```python
from build123d import *

# Parameters (mm, degrees)
F0_W     = 75.6683796644
F0_H     = 56.6312596202
F1_DEPTH = 76.2
F2_R     = 32.8805478482
F2_R_2   = 27.3422805509
F2_R_3   = 19.1504254532
F2_R_4   = 11.9146478849
F3_DEPTH = 25.4
F4_R     = 25.8365396263
F4_R_2   = 16.7772933898
F4_R_3   = 9.0542222029
F5_DEPTH = 25.4
F6_T     = -2.54
F7_R     = 3.661512341
F7_R_2   = 9.1001332581
F7_R_3   = 2.6513181401
F7_R_4   = 8.8835137034
F7_R_5   = 3.3715323173
F7_R_6   = 9.593089253
F7_R_7   = 4.4394708986
F7_R_8   = 7.7443328278
F7_R_9   = 7.7443291059
F8_DEPTH = 25.4


with BuildPart() as f1:
    # F0 (on Front) → F1 (new body)
    with BuildSketch(Plane.XZ):
        with Locations((37.8341898322, 28.3156298101)):
            Rectangle(F0_W, F0_H)
    extrude(amount=F1_DEPTH)

    # F2 (on face) → F3 (join)
    with BuildSketch(Plane.XY.offset(56.6312596202)):
        with Locations((41.328176856, -39.9102717638)):
            Circle(F2_R)
        with Locations((41.328176856, -39.9102717638)):
            Circle(F2_R_2, mode=Mode.SUBTRACT)
        with Locations((41.328176856, -39.9102717638)):
            Circle(F2_R_2)
        with Locations((41.328176856, -39.9102717638)):
            Circle(F2_R_3, mode=Mode.SUBTRACT)
        with Locations((41.328176856, -39.9102717638)):
            Circle(F2_R_4)
    extrude(amount=F3_DEPTH)

    # F4 (on face) → F5 (join)
    with BuildSketch(Plane(origin=(0, 0, 0), x_dir=(0, -1, 0), z_dir=(-1, 0, 0))):
        with Locations((38.5897643864, 28.854271397)):
            Circle(F4_R)
        with Locations((38.5897643864, 28.854271397)):
            Circle(F4_R_2, mode=Mode.SUBTRACT)
        with Locations((38.5897643864, 28.854271397)):
            Circle(F4_R_2)
        with Locations((38.5897643864, 28.854271397)):
            Circle(F4_R_3, mode=Mode.SUBTRACT)
        with Locations((38.5897643864, 28.854271397)):
            Circle(F4_R_3)
    extrude(amount=F5_DEPTH)

    # F6
    f6_openings = [f1.faces().sort_by_distance(p)[0] for p in [
        (37.83419, -76.2, 28.31563),
    ]]
    offset(amount=F6_T, openings=f6_openings, kind=Kind.INTERSECTION)

    # F7 (on face) → F8 (join)
    with BuildSketch(Plane.YZ.offset(75.6683796644)):
        with Locations((-8.7984241545, 43.9281985164)):
            Circle(F7_R)
        with Locations((-25.612493977, 40.552649647)):
            Circle(F7_R_2)
        with Locations((-40.1582121849, 43.9281985164)):
            Circle(F7_R_3)
        with Locations((-42.6249019802, 32.3069766164)):
            Circle(F7_R_4)
        with Locations((-43.8523180783, 17.5502598286)):
            Circle(F7_R_5)
        with Locations((-27.9581807554, 16.7665481567)):
            Circle(F7_R_6)
        with Locations((-15.7014150172, 29.2281731963)):
            Circle(F7_R_7)
        with BuildLine():
            Line((0, 7.6459474177), (0, 12.9123390406))
            ThreePointArc((0, 12.9123390406), (-10.0560886873, 10.2791432291), (0, 7.6459474177))
        make_face()
        with Locations((-64.4422322512, 47.1135601401)):
            Circle(F7_R_8)
        with Locations((-64.5220428705, 12.6286838204)):
            Circle(F7_R_9)
    extrude(amount=F8_DEPTH)


solid = f1.part
```
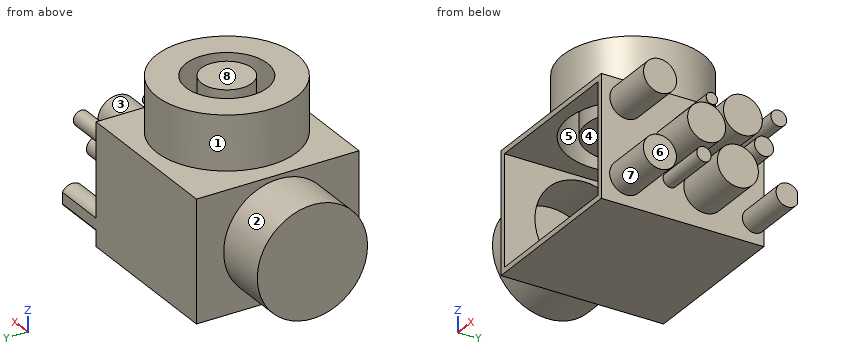
Model file for the job. Use its own axes, mm. Face numbers are marked on the shaded views. A direction names the side the tool comes from. Coordinates: 2 decimals unless noted, no trailing zeros. Loops run counter-clockwise (first coordinate to the right, second up) from the corner with the lowest first, then second, coordinate; pieces in that order, holes last. Notation, with made-up numbers: (57.5, -36) - (99.5, -36) arc R17 cw to (99.5, -10) - close; hole circle Ø7 at (-22, -1.5). An arc over 180 degrees is marked (long way). Answer as a JSON object with one key per item and string values. Group by question number.
(1) Tool access for the marked faces 1, 2, 3, 4 and 5: list every direction of +Z, -Z, +X, -X, +Y, -Y with a clear straight run to the whole face (end or side of a thin tool).
(2) Probe line 1 along X through (y, z) = (-47.5, 45.5); line 2 along X through (y, z) = (-20.5, 77); line 3 along Z through (x, y) = (43.5, -35.5). List the from-to ranges inside material, lowest first.
(3) Cut at D-D (z = 36.5). Give the cut face in (x, y).
(4) Flat gauge pins, fed straight in: pin 1 (12 mm diameter, centred on x = 68, y = -59.5, fed in from -Z); pin 2 (5 mm diameter, centred on x = 1, y = -45, fed in from +Z); pin 3 (1 mm diameter, centred on y = -42, z = 51, fed in from +X); pin 4 (1 mm diameter, centred on y = -20, z = 68.5, fed in from -X). Where does each tip first touch, or does it go through?
(5) Cut at B-B (x = 55). Give the cut face in (y, z), then the cut area to 3 significant figures.
(6) Cut at C-C (x = 81.5). State how many separate pieces and enclosed holes the cut face has, then the cut area to 3 significant figures.
(7) Cut at A-A (z = 66.5). Give the cut face in (x, y).
(8) Two-plate mould, pull along Z, no slides. Class the marked faces 6, 7 and 8: released by +Z, released by -Z, zero draft, split by the parting line, or undercut.
Geometry says:
{
 "1": {"face 1": "+Z", "face 2": "-X", "face 3": "+X", "face 4": "-Y", "face 5": "none"},
 "2": {"line 1": "x = -25.4 to -22.86, 73.13 to 75.67", "line 2": "x = 14.79 to 18.01, 31.65 to 51.01, 64.65 to 67.87", "line 3": "z = 0 to 2.54, 79.49 to 82.03"},
 "3": {"outline": "(-25.4, -63.27) - (0, -63.27) - (0, -76.2) - (2.54, -76.2) - (2.54, -60.6) - (-22.86, -60.6) - (-22.86, -16.58) - (2.54, -16.58) - (2.54, -2.54) - (73.13, -2.54) - (73.13, -76.2) - (75.67, -76.2) - (75.67, -50.46) - (101.07, -50.46) - (101.07, -34.79) - (75.67, -34.79) - (75.67, -33.76) - (101.07, -33.76) - (101.07, -17.46) - (75.67, -17.46) - (75.67, 0) - (0, 0) - (0, -13.91) - (-25.4, -13.91) - close"},
 "4": {"pin 1": "stops at z = 0", "pin 2": "stops at z = 56.63", "pin 3": "stops at x = 75.67", "pin 4": "stops at x = 14.79"},
 "5": {"outline": "(-76.2, 0) - (0, 0) - (0, 56.63) - (-10.01, 56.63) - (-10.01, 82.03) - (-26.5, 82.03) - (-26.5, 56.63) - (-53.32, 56.63) - (-53.32, 82.03) - (-69.81, 82.03) - (-69.81, 56.63) - (-76.2, 56.63) - (-76.2, 54.09) - (-67, 54.09) - (-67, 79.49) - (-56.75, 79.49) - (-56.75, 54.09) - (-23.07, 54.09) - (-23.07, 79.49) - (-12.82, 79.49) - (-12.82, 54.09) - (-2.54, 54.09) - (-2.54, 2.54) - (-76.2, 2.54) - close", "area": "835 mm^2"},
 "6": {"separate pieces": "10", "enclosed holes": "0", "area": "1,420 mm^2"},
 "7": {"outline": "circle Ø65.76 at (41.33, -39.91); circle Ø43.38 at (41.33, -39.91); circle Ø23.83 at (41.33, -39.91); hole circle Ø60.68 at (41.33, -39.91); hole circle Ø38.3 at (41.33, -39.91); hole circle Ø18.75 at (41.33, -39.91)"},
 "8": {"face 6": "zero draft", "face 7": "undercut", "face 8": "released by +Z"}
}
